Geometry check sheet. Reference: the model listing, model coordinates, mm. A direction names the side the tool comes from. Give positions to 0.01 mm unless a question says otherwise; leave off trailing zeros. Write each loop counter-clockwise with the first axis right and the second up, starting at its lowest first coordinate (ties: lowest second). Pieces come first, ordered by that corner, then holes. Notation, with made-up numbers: (-26, 71) - (24, 71) arc R25 ccw to (24, 85) - close; hole circle Ø5 at (59, -6.5). An arc over 180 degrees is marked (long way). Use a Markdown table: item, result.
```python
from build123d import *

# Parameters (mm, degrees)
F1_DEPTH = 16
F2_R     = 3.7
F3_DEPTH = 22
F4_DEPTH = 21
F6_D     = 4.5


with BuildPart() as f1:
    # F0 (on Front) → F1 (new body)
    with BuildSketch(Plane.XZ):
        Polygon((0.202192, 32.007239), (-12.797808, 32.007239), (-12.797808, 19.507239), (-12.797808, -8.492761), (-12.797808, -26.992761), (0.202192, -26.992761), align=None)
    extrude(amount=F1_DEPTH)

    # F2 (on face) → F3 (join)
    with BuildSketch(Plane(origin=(-12.797808, 0, 0), x_dir=(0, -1, 0), z_dir=(-1, 0, 0))):
        with Locations((7.996093, 26.00724)):
            Circle(F2_R)
    extrude(amount=F3_DEPTH)

    # F2 (on face) → F4 (join)
    with BuildSketch(Plane(origin=(-12.797808, 0, 0), x_dir=(0, -1, 0), z_dir=(-1, 0, 0))):
        with Locations((8, -19.492761)):
            Circle(F2_R)
    extrude(amount=F4_DEPTH)

    # F6 (through all)
    with Locations(Plane.YZ.offset(0.202192)):
        with Locations((-7.788272, 2.507239)):
            Hole(F6_D / 2)


solid = f1.part
```
1) Depth check by flat-ended pin: P1, Ø3.5, axis at y = -9, z = -18, coming from the -X side; P2, Ø4, axis at y = -7.79, z = 2.51, coming from the +X side; P3, Ø2, axis at y = -3.5, z = 22, coming from the -X side. Enter the tip coordinate at first touch or a pass-through.
Working result:
| item | result |
|---|---|
| P1 | stops at x = -33.8 |
| P2 | passes through |
| P3 | stops at x = -12.8 |
2) Section check D-D on y = -11. Record the boundary of the cut face in (x, z).
Working result:
| item | result |
|---|---|
| outline | (-34.8, 23.85) - (-12.8, 23.85) - (-12.8, -17.33) - (-33.8, -17.33) - (-33.8, -21.66) - (-12.8, -21.66) - (-12.8, -26.99) - (0.2, -26.99) - (0.2, 32.01) - (-12.8, 32.01) - (-12.8, 28.17) - (-34.8, 28.17) - close |
3) Material ranges on L1, parallel to X at y = -14.25, z = -19; L2, parallel to Z at x = -21, y = -6.75; L3, parallel to Z at x = -20, y = -6, recorded low to high. Write a range as from..to.
Working result:
| item | result |
|---|---|
| L1 | x = -12.8..0.2 |
| L2 | z = -22.98..-16.01, 22.52..29.49 |
| L3 | z = -22.61..-16.38, 22.89..29.12 |
4) Section check A-A on y = -7.25. Record the boundary of the cut face in (x, z), then the cut area to 3 significant figures.
Working result:
| item | result |
|---|---|
| outline | (-34.8, 22.38) - (-12.8, 22.38) - (-12.8, 4.69) - (0.2, 4.69) - (0.2, 32.01) - (-12.8, 32.01) - (-12.8, 29.63) - (-34.8, 29.63) - close; (-33.8, -23.12) - (-12.8, -23.12) - (-12.8, -26.99) - (0.2, -26.99) - (0.2, 0.32) - (-12.8, 0.32) - (-12.8, -15.87) - (-33.8, -15.87) - close |
| area | 1,020 mm² |
5) Section check B-B on z = 1.5. Record the boundary of the cut face in (x, y).
Working result:
| item | result |
|---|---|
| outline | (-12.8, -16) - (0.2, -16) - (0.2, -9.8) - (-12.8, -9.8) - close; (-12.8, -5.78) - (0.2, -5.78) - (0.2, 0) - (-12.8, 0) - close |
6) Section check C-C on z = 23. Record the boundary of the cut face in (x, y).
Working result:
| item | result |
|---|---|
| outline | (-34.8, -10.15) - (-12.8, -10.15) - (-12.8, -16) - (0.2, -16) - (0.2, 0) - (-12.8, 0) - (-12.8, -5.84) - (-34.8, -5.84) - close |
7) Set-up check for faces 1 (the flat face through (-34.798, -8, 26)), 2 (the flat face through (-33.798, -8, -19)), 3 (the flat face through (-12.798, -11, 3)): record each of +Z, -Z, +X, -X, +Y, -Y from which the full face is reachable in a straight line by a thin tool's end or side.
Working result:
| item | result |
|---|---|
| face 1 | +Z, -Z, -X, +Y, -Y |
| face 2 | -Z, -X, +Y, -Y |
| face 3 | -X |
